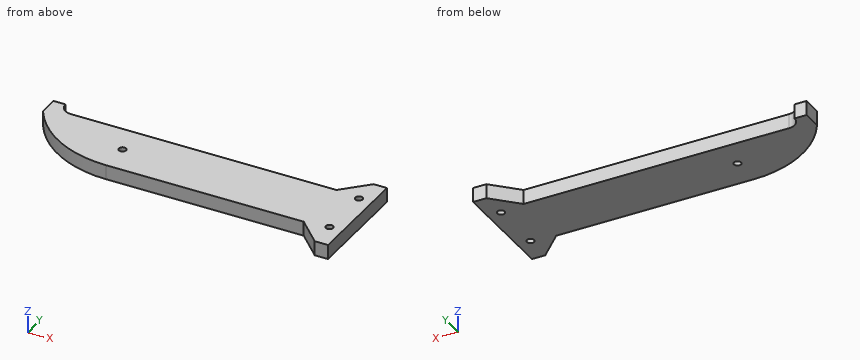
```python
from build123d import *

# Parameters (mm, degrees)
SKETCH1_R           = 1.5
BOSS_EXTRUDE1_DEPTH = 6


with BuildPart() as part:
    # Sketch1 → Boss-Extrude1 (new body)
    with BuildSketch(Plane.XY):
        with BuildLine():
            Line((120, -25), (38.105117767, -25))
            ThreePointArc((38.105117767, -25), (16.105117767, -19.105117767), (0, -3))
            Line((0, -3), (0, 0))
            Line((0, 0), (0, 5))
            Line((0, 5), (5, 5))
            ThreePointArc((5, 5), (6.464466094, 1.464466094), (10, 0))
            Line((10, 0), (120, 0))
            Line((120, 0), (130, 10))
            Line((130, 10), (135.5, 10))
            Line((135.5, 10), (135.5, -35))
            Line((135.5, -35), (130, -35))
            Line((130, -35), (120, -25))
        make_face()
        with Locations((130, -1.25)):
            Circle(SKETCH1_R, mode=Mode.SUBTRACT)
        with Locations((130, -23.75)):
            Circle(SKETCH1_R, mode=Mode.SUBTRACT)
        with Locations((38.105117767, -12.5)):
            Circle(SKETCH1_R, mode=Mode.SUBTRACT)
    extrude(amount=BOSS_EXTRUDE1_DEPTH)


solid = part.part
```
The model under review builds one solid part; all positions refer to its coordinate system, in mm. Round coordinates to 2 decimals unless told otherwise and drop trailing zeros. Write each loop counter-clockwise with the first axis right and the second up, starting at its lowest first coordinate (ties: lowest second). Pieces come first, ordered by that corner, then holes.
(1) We need section D-D on x = 76. Give the boundary of the cut face in (y, z), and give its area (3 significant figures).
(2) Wall thickness on L1, parallel to Y at x = 130, z = 2.6; L2, parallel to X at y = 0.5, z = 1; L3, parallel to Y at x = 101.5, z = 3.5: over which ranges is each line inside the solid? List them lowest first.
(3) We need section C-C on y = -23.75. Give the boundary of the cut face in (x, z).
(4) Insertion check: pin 1 (2 mm diameter, centred on x = 79, z = 3.5, fed in from +Y); pin 2 (3 mm diameter, centred on x = 84, z = 3, fed in from -Y). Each pin has a flat end and moves straight along its axis. Give the tip position at first contact, or say it passes through.
(5) We need section A-A on y = -1.25. Give the boundary of the cut face in (x, z), and give its area (3 significant figures).
(6) We need section B-B on z = 1.95. Give the boundary of the cut face in (x, y).
Findings below:
1. outline: (-25, 0) - (0, 0) - (0, 6) - (-25, 6) - close
1. area: 150 mm2
2. L1: y = -35 to -25.25, -22.25 to -2.75, 0.25 to 10
2. L2: x = 0 to 7.82, 120.5 to 135.5
2. L3: y = -25 to 0
3. outline: (27.69, 0) - (128.5, 0) - (128.5, 6) - (27.69, 6) - close; (131.5, 0) - (135.5, 0) - (135.5, 6) - (131.5, 6) - close
4. pin 1: stops at y = 0
4. pin 2: stops at y = -25
5. outline: (0, 0) - (128.5, 0) - (128.5, 6) - (0, 6) - close; (131.5, 0) - (135.5, 0) - (135.5, 6) - (131.5, 6) - close
5. area: 795 mm2
6. outline: (0, -3) arc R44 ccw to (38.11, -25) - (120, -25) - (130, -35) - (135.5, -35) - (135.5, 10) - (130, 10) - (120, 0) - (10, 0) arc R5 cw to (5, 5) - (0, 5) - close; hole circle Ø3 at (38.11, -12.5); hole circle Ø3 at (130, -23.75); hole circle Ø3 at (130, -1.25)
